from build123d import *

# Parameters (mm, degrees)
SKETCH1_W                       = 317.5
SKETCH1_H                       = 317.5
SKETCH1_R                       = 15.875
BOSS_EXTRUDE1_DEPTH             = 25.4
F_3_4_0_75_DIAMETER_HOLE2_D     = 19.05
F_3_4_0_75_DIAMETER_HOLE2_DEPTH = 76.2
F_3_4_0_75_DIAMETER_HOLE2_TIP   = 5.723197396
F_3_4_0_75_DIAMETER_HOLE1_D     = 19.05
F_3_4_0_75_DIAMETER_HOLE1_DEPTH = 76.2
F_3_4_0_75_DIAMETER_HOLE1_TIP   = 5.723197396


with BuildPart() as part:
    # Sketch1 → Boss-Extrude1 (new body)
    with BuildSketch(Plane(origin=(0, 0, 0), x_dir=(1, 0, 0), z_dir=(0, 1, 0))):
        Rectangle(SKETCH1_W, SKETCH1_H)
        Circle(SKETCH1_R, mode=Mode.SUBTRACT)
    extrude(amount=BOSS_EXTRUDE1_DEPTH)

    # 3/4 (0.75) Diameter Hole2
    with Locations(Plane(origin=(158.75, 0, 0), x_dir=(0, 0, -1), z_dir=(1, 0, 0))):
        with Locations((0, 12.7)):
            Hole(F_3_4_0_75_DIAMETER_HOLE2_D / 2, depth=F_3_4_0_75_DIAMETER_HOLE2_DEPTH)
            with Locations((0, 0, -(F_3_4_0_75_DIAMETER_HOLE2_DEPTH + F_3_4_0_75_DIAMETER_HOLE2_TIP / 2))):  # 118° drill point
                Cone(0, F_3_4_0_75_DIAMETER_HOLE2_D / 2, F_3_4_0_75_DIAMETER_HOLE2_TIP, mode=Mode.SUBTRACT)

    # 3/4 (0.75) Diameter Hole1
    with Locations(Plane.XY.offset(158.75)):
        with Locations((0, 12.7)):
            Hole(F_3_4_0_75_DIAMETER_HOLE1_D / 2, depth=F_3_4_0_75_DIAMETER_HOLE1_DEPTH)
            with Locations((0, 0, -(F_3_4_0_75_DIAMETER_HOLE1_DEPTH + F_3_4_0_75_DIAMETER_HOLE1_TIP / 2))):  # 118° drill point
                Cone(0, F_3_4_0_75_DIAMETER_HOLE1_D / 2, F_3_4_0_75_DIAMETER_HOLE1_TIP, mode=Mode.SUBTRACT)


solid = part.part
Verification items for the finished model (mm, model axes). A direction names the side the tool comes from. Round coordinates to 2 decimals unless told otherwise and drop trailing zeros. Loops run counter-clockwise (first coordinate to the right, second up) from the corner with the lowest first, then second, coordinate; pieces in that order, holes last. Notation, with made-up numbers: (81.5, -37.75) - (132.5, -37.75) arc R32 ccw to (132.5, -8.75) - close; hole circle Ø11 at (-33.75, 74.25). An arc over 180 degrees is marked (long way). Use one line per item in the form item = value.
1. Scan lines: probe 1 along Z at (x, y) = (124, 12.7) (3 decimals); probe 2 along Y at (x, z) = (0, 122) (3 decimals). Record each from-to range of solid material in increasing order.
A:
probe_1 = -158.75 to -9.525, 9.525 to 158.75
probe_2 = 0 to 3.175, 22.225 to 25.4
2. Draft check along Z on faces 1 (the cylindrical face through (-3.441, 12.522, 15.497)), 2 (the flat face through (-2, 13, -158.75)), 3 (the flat face through (-158.75, 13, 2)). Enter one of: pulls with the +Z half, pulls with the -Z half, needs draft (parallel to the pull), parting line crosses it, or undercut.
A:
face_1 = undercut
face_2 = pulls with the -Z half
face_3 = needs draft
3. Section check B-B on x = 109. Record the cut outline in (y, z) (3 decimals).
A:
outline = (0, -158.75) - (25.4, -158.75) - (25.4, 158.75) - (0, 158.75) - close; hole circle Ø19.05 at (12.7, 0)
4. Section check A-A on z = 127.5. Record the cut outline in (x, y) (3 decimals), and give its area (3 significant figures).
A:
outline = (-158.75, 0) - (158.75, 0) - (158.75, 25.4) - (-158.75, 25.4) - close; hole circle Ø19.05 at (0, 12.7)
area = 7,780 mm²
5. Access from +Z, -Z, +X, -X, +Y, -Y to the whole of each face (thin tool, end or side, straight path). Record for faces 4 (the cylindrical face through (120.12, 3.4, -2.06)), 5 (the flat face through (-2, 0, -38)), 6 (the cylindrical face through (2.06, 3.4, 120.12)).
A:
face_4 = +X
face_5 = +Z, -Z, +X, -X, -Y
face_6 = +Z
